The listing builds one solid part. Answer for the finished solid, in the listing's coordinates (mm). Face numbers are marked on the shaded views. A direction names the side the tool comes from. Coordinates: 2 decimals unless noted, no trailing zeros. Order: outer loops, then holes, each group sorted by start corner. A loop starts at its lowest first (then second) coordinate and runs counter-clockwise, first axis right, second up.
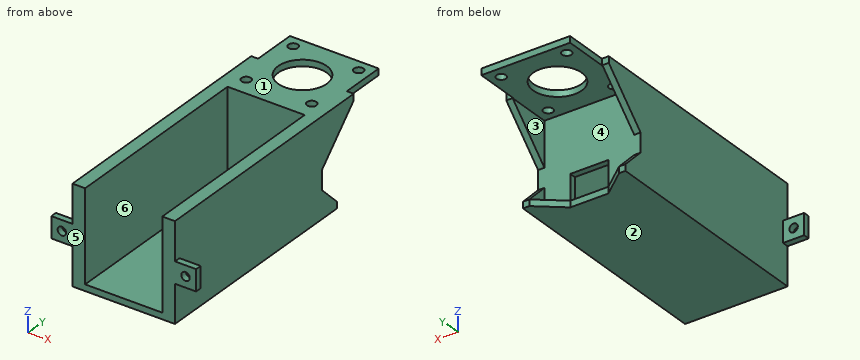
Autodesk Inventor part; units mm, degrees
ref_plane "YZ Plane" through (0, 0, 0) normal (1, 0, 0) x (0, 1, 0)
ref_plane "XZ Plane" through (0, 0, 0) normal (0, 1, 0) x (-1, 0, 0)
ref_plane "XY Plane" through (0, 0, 0) normal (0, 0, 1) x (1, 0, 0)
sketch "Boceto1" plane through (0, 0, 0) normal (0, 0, 1) x (1, 0, 0)
  line L0 (-21, 21) -> (21, 21)
  line L1 (21, 21) -> (21, -21)
  line L2 (21, -21) -> (-21, -21)
  line L3 (-21, -21) -> (-21, 21)
  circle A0 centre (0, 0) radius 11.5
  circle A1 centre (-15.5, 15.5) radius 2.25
  circle A2 centre (-15.5, -15.5) radius 2.25
  circle A3 centre (15.5, -15.5) radius 2.25
  circle A4 centre (15.5, 15.5) radius 2.25
  dimension "d0" = 42
  dimension "d1" = 42
  dimension "d2" = 23
  dimension "d6" = 4.5
  dimension "d7" = 4.5
  dimension "d8" = 4.5
  dimension "d9" = 4.5
extrude "Extrusión1" add sketch "Boceto1" along normal blind 3
sketch "Boceto28" plane through (0, 0, 3) normal (0, 0, 1) x (1, 0, 0)
  line L0 (-21.25, -24) -> (21.25, -24)
  line L1 (21.25, -24) -> (21.25, -21)
  line L2 (-21.25, -21) -> (-21.25, -24)
  line L3 (-21, -21) -> (21, -21)
  line L4 (21.25, -21) -> (-21.25, -21)
  point P0 (0, 0)
extrude "Extrusión24" add sketch "Boceto28" against normal blind 43
sketch "Boceto29" plane through (-21.25, -21, -40) normal (0, 1, 0) x (1, 0, 0)
  line L0 (30.25, -12) -> (12.25, -12)
  line L1 (0, 0) -> (42.5, 0)
  line L2 (12.25, 0) -> (30.25, 0)
  line L3 (12.25, 0) -> (12.25, -12)
  line L4 (30.25, 0) -> (30.25, -12)
  point P0 (21.25, -40)
extrude "Extrusión25" cut sketch "Boceto29" against normal blind 3
sketch "Boceto33" plane through (21.25, -24, 3) normal (1, 0, 0) x (0, 0, -1)
  line L0 (43, 0) -> (33, 0)
  line L1 (33, 0) -> (33, 3)
  line L2 (43, 0) -> (46, 0)
  line L3 (46, 0) -> (46, 13)
  line L4 (46, 13) -> (43, 13)
  line L5 (43, 13) -> (33, 3)
  line L6 (0, 45) -> (0, 3)
  line L7 (0, 0) -> (43, 0)
  line L8 (0, 24) -> (0, 0)
  line L9 (0, 0) -> (24, 0)
  line L10 (24, 0) -> (24, 3)
  line L11 (0, 3) -> (43, 3)
  line L12 (0, 24) -> (3, 24)
  line L13 (3, 45) -> (3, 3)
  line L14 (3, 24) -> (24, 3)
  point P0 (0, 3)
  dimension "d153" = 10
  dimension "d154" = 3
  dimension "d155" = 13
  dimension "d156" = 3
  dimension "d181" = 24
extrude "Extrusión28" add sketch "Boceto33" along normal blind 3 contours L0 L1 L5 L4 L3 L2 | L7 L8 L11 L10 | L11 L13 L14 | L11 L6 L12 L13
sketch "Boceto34" plane through (-21.25, -24, 3) normal (-1, 0, 0) x (0, 0, 1)
  line L0 (-46, 0) -> (-46, 13)
  line L1 (-46, 13) -> (-43, 13)
  line L2 (-46, 13) -> (-43, 13)
  line L3 (-43, 13) -> (-33, 3)
  line L4 (-43, 0) -> (-46, 0)
  line L5 (-46, 13) -> (-46, 0)
  line L6 (-46, 0) -> (-33, 0)
  line L7 (-33, 3) -> (-33, 0)
  line L8 (-24, 0) -> (-24, 3)
  line L9 (-24, 3) -> (-3, 24)
  line L10 (0, 24) -> (-3, 24)
  line L11 (-24, 0) -> (0, 0)
  line L12 (0, 0) -> (0, 24)
extrude "Extrusión29" add sketch "Boceto34" along normal blind 3
sketch "Boceto36" plane through (0, 0, -40) normal (0, 0, -1) x (-1, 0, 0)
  line L0 (9, -21) -> (9, -24)
  line L1 (9, -24) -> (21.25, -24)
  line L2 (21.25, -24) -> (21.25, -11)
  line L3 (9, -21) -> (9, -24)
  line L4 (-9, -24) -> (-9, -21)
  line L5 (-9, -21) -> (-9, -24)
  line L6 (-21, -21) -> (-21, 21)
  line L7 (-21.25, -11) -> (-9, -21)
  line L8 (-21.25, -11) -> (-21.25, -24)
  line L9 (24.25, -24) -> (-24.25, -24)
  line L10 (-9, -24) -> (-21.25, -24)
  line L11 (9, -21) -> (21.25, -11)
extrude "Extrusión31" add sketch "Boceto36" along normal blind 3
sketch "Boceto37" plane through (-21, -21, 0) normal (0, 1, 0) x (1, 0, 0)
  line L0 (45.25, 40) -> (45.25, 30)
  line L1 (42.25, 21) -> (42.25, 0)
  line L2 (45.25, 30) -> (42.25, 30)
  line L3 (42.25, 30) -> (42.25, 21)
  line L4 (42.25, 21) -> (45.25, 21)
  line L5 (45.25, 21) -> (45.25, 30)
  line L6 (30, 40) -> (30, 43)
  line L7 (12, 43) -> (12, 28)
  line L8 (30, 40) -> (12, 40)
  line L9 (12, 40) -> (12, 43)
  line L10 (12, 43) -> (30, 43)
  line L11 (30, 43) -> (30, 40)
  line L12 (-0.25, 21) -> (-0.25, 30)
  line L13 (-3.25, 0) -> (-3.25, 21)
  line L14 (-0.25, 30) -> (-3.25, 30)
  line L15 (-3.25, 30) -> (-3.25, 21)
  line L16 (-3.25, 21) -> (-0.25, 21)
  line L17 (-0.25, 21) -> (-0.25, 30)
extrude "Extrusión32" add sketch "Boceto37" against normal blind 3
sketch "Boceto38" plane through (0, 0, 3) normal (0, 0, 1) x (1, 0, 0)
  line L0 (-21.25, 0) -> (-21.25, -21)
  line L1 (-21, -21) -> (-21.25, -21)
  line L2 (-21.25, 0) -> (-21, 0)
  line L3 (-21, 0) -> (-21, -21)
  line L4 (-21, -21) -> (-21.25, -21)
  line L5 (-21.25, -21) -> (-21.25, 0)
  line L6 (21, -21) -> (21, 21)
  line L7 (21.25, 0) -> (21.25, -21)
  line L8 (21, -21) -> (21.25, -21)
  line L9 (21.25, -21) -> (21.25, 0)
  line L10 (21.25, 0) -> (21, 0)
  line L11 (21, 0) -> (21, -21)
extrude "Extrusión33" add sketch "Boceto38" against normal blind 3
sketch "Boceto50" plane through (24.25, -24, -43) normal (0, -1, 0) x (1, 0, 0)
  line L0 (-45.5, 0) -> (-48.5, 0)
  line L1 (-48.5, 0) -> (-48.5, 46)
  line L2 (-48.5, 0) -> (-48.5, 46)
  line L3 (-48.5, 46) -> (-42.5, 46)
  line L4 (-42.5, 46) -> (-42.5, 3)
  line L5 (-48.5, 0) -> (0, 0)
  line L6 (-48.5, 0) -> (0, 0)
  line L7 (0, 0) -> (0, 46)
  line L8 (0, 46) -> (-6, 46)
  line L9 (-6, 46) -> (-6, 3)
  line L10 (-42.5, 3) -> (-6, 3)
  dimension "d183" = 6
  dimension "d184" = 6
extrude "Extrusión39" add sketch "Boceto50" along normal blind 94
sketch "Boceto51" plane through (24.25, -24, 3) normal (1, 0, 0) x (0, 0, -1)
  line L0 (18, -94) -> (28, -94)
  line L1 (28, -94) -> (28, -91)
  line L2 (28, -91) -> (18, -91)
  line L3 (18, -91) -> (18, -94)
  point P0 (3, 24)
  dimension "d171" = 10
  dimension "d172" = 3
extrude "Extrusión40" add sketch "Boceto51" along normal blind 10
sketch "Boceto52" plane through (-24.25, -24, 3) normal (-1, 0, 0) x (0, 0, 1)
  line L0 (0, -94) -> (-46, -94)
  line L1 (-18, -91) -> (-18, -94)
  line L2 (-23, -94) -> (-18, -94)
  line L3 (-18, -94) -> (-18, -91)
  line L4 (-28, -91) -> (-18, -91)
  line L5 (-18, -91) -> (-28, -91)
  line L6 (-28, -94) -> (-28, -91)
  line L7 (-28, -91) -> (-28, -94)
  line L8 (-28, -94) -> (-23, -94)
  point P0 (-3, 24)
extrude "Extrusión41" add sketch "Boceto52" along normal blind 10
sketch "Boceto56" plane through (-24.25, -115, -15) normal (0, 1, 0) x (1, 0, 0)
  line L0 (48.5, 0) -> (58.5, 0)
  line L1 (48.5, 10) -> (58.5, 10)
  line L2 (0, 10) -> (-10, 10)
  line L3 (0, 0) -> (-10, 0)
  line L4 (-10, 0) -> (-10, 10)
  circle A0 centre (-5, 5) radius 2
  circle A1 centre (53.5, 5) radius 2
  point P0 (24.25, -15)
  dimension "d185" = 4
  dimension "d186" = 4
extrude "Extrusión43" cut sketch "Boceto56" against normal blind 3
properties part number "Torre Motor Definitiva" material "Plástico ABS"
1) Each of these flat-tipped pins is pushed along its axis until it touches: P1, Ø2.5, axis at x = -22.5, z = 1.5, coming from the +Y side; P2, Ø1.5, axis at y = -22.5, z = -32.5, coming from the -X side; P3, Ø3.5, axis at y = -23, z = -31.5, coming from the +X side; P4, Ø3, axis at x = -29.25, z = -20, coming from the +Y side. Where does it stop, or does it pass through?
2) Section B-B (y = 15.5) is taken. Give the vertices of the cut face in (x, z), then the cut area to 3 significant figures.
3) Section C-C (x = 4.5) is taken. Give the vertices of the cut face in (y, z), then the cut area to 3 significant figures.
4) A tool of negligible diameter and unlimited length cuts with its end or side. For the marked faces 4, 5 and 6, from which of +Z, -Z, +X, -X, +Y, -Y can it reach the whole face along a straight path? Write none if from no direction.
5) Section D-D (z = -10) is taken. Give the vertices of the cut face in (x, y), then the cut area to 3 significant figures.
6) Section A-A (z = -32.5) is taken. Give the vertices of the cut face in (x, y).
7) Consider L1, parallel to Y at x = -15.5, z = 1.65; L2, parallel to X at y = -106.5, z = 0; L3, parallel to Z at x = 12, y = -19. Determine where each line is inside the solid, lowest interval first.
8) Determine the mould class of the marked faces 1, 2 and 3 for opening direction Z: released by +Z, released by -Z, zero draft, split by the parting line, or undercut.
Filled sheet:
1. P1: stops at y = 0
1. P2: stops at x = -24.25
1. P3: stops at x = 24.25
1. P4: passes through
2. outline: (-21, 0) - (-17.75, 0) - (-17.75, 3) - (-21, 3) - close; (-13.25, 0) - (13.25, 0) - (13.25, 3) - (-13.25, 3) - close; (17.75, 0) - (21, 0) - (21, 3) - (17.75, 3) - close
2. area: 99.0 mm2
3. outline: (-118, -43) - (-21, -43) - (-21, -40) - (-118, -40) - close; (-24, -28) - (-21, -28) - (-21, 0) - (-10.58, 0) - (-10.58, 3) - (-24, 3) - close; (10.58, 0) - (21, 0) - (21, 3) - (10.58, 3) - close
3. area: 447 mm2
4. face 4: +Y
4. face 5: +Z, -Z, +X, -X, -Y
4. face 6: +Z, -Y
5. outline: (-24.25, -118) - (-18.25, -118) - (-18.25, -24) - (18.25, -24) - (18.25, -118) - (24.25, -118) - (24.25, -10) - (21.25, -10) - (21.25, -21) - (-21.25, -21) - (-21.25, -10) - (-24.25, -10) - close
5. area: 1,340 mm2
6. outline: (-24.25, -118) - (-18.25, -118) - (-18.25, -24) - (-9, -24) - (-9, -21) - (-21.25, -21) - (-21.25, -18.5) - (-24.25, -18.5) - close; (9, -24) - (18.25, -24) - (18.25, -118) - (24.25, -118) - (24.25, -18.5) - (21.25, -18.5) - (21.25, -21) - (9, -21) - close
7. L1: y = -24 to -17.75, -13.25 to 13.25, 17.75 to 21
7. L2: x = -24.25 to -18.25, 18.25 to 24.25
7. L3: z = -43 to -40, 0 to 3
8. face 1: released by +Z
8. face 2: released by -Z
8. face 3: undercut
